```python
from build123d import *

# Parameters (mm, degrees)
SKETCH1_W               = 177.8
SKETCH1_H               = 50.8
BOSS_EXTRUDE1_DEPTH     = 3.175
SKETCH2_W               = 3.175
SKETCH2_H               = 50.8
BOSS_EXTRUDE2_DEPTH     = 63.5
FILLET1_R               = 6.35
F_1_0MM_DOWEL_HOLE1_D   = 4.318
F_1_0MM_DOWEL_HOLE2_D   = 12.7
ADVANCEDHOLE1_OUTLINE_R = 2.159
ADVANCEDHOLE1_DEPTH     = 3.175


# Read off the part's stored shape, not the designer's step: AdvancedHole1
with BuildPart() as part:
    # Sketch1 → Boss-Extrude1 (new body)
    with BuildSketch(Plane(origin=(0, 0, 0), x_dir=(1, 0, 0), z_dir=(0, 1, 0))):
        Rectangle(SKETCH1_W, SKETCH1_H)
    extrude(amount=BOSS_EXTRUDE1_DEPTH)

    # Sketch2 → Boss-Extrude2 (add)
    with BuildSketch(Plane(origin=(0, 3.175, 0), x_dir=(1, 0, 0), z_dir=(0, 1, 0))):
        with Locations((-87.3125, 0)):
            Rectangle(SKETCH2_W, SKETCH2_H)
    extrude(amount=BOSS_EXTRUDE2_DEPTH)

    # Fillet1
    fillet1_edges = [part.edges().sort_by_distance(p)[0] for p in [
        (-85.725, 3.175, 0),
        (-88.9, 0, 0),
    ]]
    fillet(fillet1_edges, radius=FILLET1_R)

    # Ø1.0mm Dowel Hole1 (through all)
    with Locations(Plane.ZY.offset(88.9)):
        with Locations((-17.960512212, 54.971024484), (17.960512272, 54.971024484), (17.960512272, 19.05), (-17.960512212, 19.05)):
            Hole(F_1_0MM_DOWEL_HOLE1_D / 2)

    # Ø1.0mm Dowel Hole2 (through all)
    with Locations(Plane(origin=(-88.9, 37.010512242, 3e-08), x_dir=(0, 0, -1), z_dir=(-1, 0, 0))):
        with Locations((0, 0)):
            Hole(F_1_0MM_DOWEL_HOLE2_D / 2)

    # AdvancedHole1 outline → AdvancedHole1 (cut)
    with BuildSketch(Plane(origin=(0, 0, 0), x_dir=(1, 0, 0), z_dir=(0, 1, 0))):
        with Locations((-69.85, -15.875)):
            Circle(ADVANCEDHOLE1_OUTLINE_R)
        with Locations((-69.85, 15.875)):
            Circle(ADVANCEDHOLE1_OUTLINE_R)
        with Locations((82.55, 15.875)):
            Circle(ADVANCEDHOLE1_OUTLINE_R)
        with Locations((82.55, -15.875)):
            Circle(ADVANCEDHOLE1_OUTLINE_R)
    extrude(amount=ADVANCEDHOLE1_DEPTH, mode=Mode.SUBTRACT)


solid = part.part
```
Input: part model. Units: mm. Frame: model coordinates. A direction names the side the tool comes from. Round coordinates to 2 decimals unless told otherwise and drop trailing zeros. Loops run counter-clockwise (first coordinate to the right, second up) from the corner with the lowest first, then second, coordinate; pieces in that order, holes last. Notation, with made-up numbers: (-21.75, 58) -> (20.25, 58) arc R24 ccw to (20.25, 80) -> close; hole circle Ø5 at (20, -31.5). An arc over 180 degrees is marked (long way). One line per item, written item: value.
(1) Material intervals for line 1 (Z direction, x = 82.55, y = 1.9); line 2 (X direction, y = 30.5, z = 13.5) (3 decimals); line 3 (Z direction, x = -69, y = 2), sorted ascending. Write a range as [from, to].
Geometry check:
line 1: [-25.4, -18.03], [-13.72, 13.72], [18.03, 25.4]
line 2: [-88.9, -85.725]
line 3: [-25.4, -17.86], [-13.89, 13.89], [17.86, 25.4]
(2) Set-up query: faces 1 (the face through (4, 3.175, 0)), 2 (the face through (-87.29, 57.11, 18.24)). Return all of +Z, -Z, +X, -X, +Y, -Y with unobstructed straight access to the full face (end or side cutting, diameter ignored); none if empty.
Geometry check:
face 1: +Z, -Z, +X, +Y
face 2: +X, -X
(3) Section A-A (z = 0). Return the cut outline in (x, y) (3 decimals), plus the area to 3 significant figures.
Geometry check:
outline: (-88.9, 6.35) arc R6.35 ccw to (-82.55, 0) -> (88.9, 0) -> (88.9, 3.175) -> (-79.375, 3.175) arc R6.35 cw to (-85.725, 9.525) -> (-85.725, 30.661) -> (-88.9, 30.661) -> close; (-88.9, 43.361) -> (-85.725, 43.361) -> (-85.725, 66.675) -> (-88.9, 66.675) -> close
area: 726 mm2
(4) Pin query (flat end, axial travel): pin 1 (12 mm diameter, centred on y = 55, z = 13.5, fed in from +X) (3 decimals); pin 2 (5 mm diameter, centred on x = -15, z = 12, fed in from +Y) (3 decimals); pin 3 (3.5 mm diameter, centred on x = 82.55, z = -15.875, fed in from +Y); pin 4 (2 mm diameter, centred on y = 9, z = 11, fed in from +X). Return the tip coordinate at first contact, or that it passes through.
Geometry check:
pin 1: x = -85.725
pin 2: y = 3.175
pin 3: through
pin 4: x = -85.54
(5) Section C-C (y = 19.05). Return the cut outline in (x, z) (3 decimals), plus the area to 3 significant figures.
Geometry check:
outline: (-88.9, -25.4) -> (-85.725, -25.4) -> (-85.725, -20.12) -> (-88.9, -20.12) -> close; (-88.9, -15.802) -> (-85.725, -15.802) -> (-85.725, 15.802) -> (-88.9, 15.802) -> close; (-88.9, 20.12) -> (-85.725, 20.12) -> (-85.725, 25.4) -> (-88.9, 25.4) -> close
area: 134 mm2
(6) Section B-B (x = 82.55). Return the cut outline in (y, z) (3 decimals).
Geometry check:
outline: (0, -25.4) -> (3.175, -25.4) -> (3.175, -18.034) -> (0, -18.034) -> close; (0, -13.716) -> (3.175, -13.716) -> (3.175, 13.716) -> (0, 13.716) -> close; (0, 18.034) -> (3.175, 18.034) -> (3.175, 25.4) -> (0, 25.4) -> close
(7) Mould query, pull axis Y, two halves, no side actions, for faces 3 (the face through (-87.09, 1.91, -0.36)), 4 (the face through (-67.79, 1.57, -16.52)), 5 (the face through (-87.29, 56.43, -16.37)). Classes: pulls with the +Y half, pulls with the -Y half, needs draft (parallel to the pull), parting line crosses it, or undercut.
Geometry check:
face 3: pulls with the -Y half
face 4: needs draft
face 5: undercut
(8) Section D-D (z = -9). Return the cut outline in (x, y) (3 decimals).
Geometry check:
outline: (-88.9, 6.35) arc R6.35 ccw to (-82.55, 0) -> (88.9, 0) -> (88.9, 3.175) -> (-79.375, 3.175) arc R6.35 cw to (-85.725, 9.525) -> (-85.725, 66.675) -> (-88.9, 66.675) -> close
